Geometry: final body of the model. Coordinates: model frame, mm. A direction names the side the tool comes from. Coordinates: 2 decimals unless noted, no trailing zeros. Write each loop counter-clockwise with the first axis right and the second up, starting at its lowest first coordinate (ties: lowest second). Pieces come first, ordered by that corner, then holes. Notation, with made-up numbers: (-23, 43) -> (-7, 43) arc R32 ccw to (-7, 71) -> close; hole circle Ø1 at (28, 86.5). An arc over 180 degrees is marked (long way). One line per item, written item: value. Start each with the question number.
from build123d import *

# Parameters (mm, degrees)
BOSS_EXTRUDE1_DEPTH = 34.75
SKETCH2_R           = 2
CUT_EXTRUDE1_DEPTH  = 72.445179815
SKETCH3_W           = 30
SKETCH3_H           = 7.896551268
BOSS_EXTRUDE2_DEPTH = 48
SKETCH4_W           = 30
SKETCH4_H           = 6
CUT_EXTRUDE2_DEPTH  = 4
FILLET1_R           = 10
SKETCH5_R           = 9
CUT_EXTRUDE3_DEPTH  = 75.652167363
BOSS_EXTRUDE3_DEPTH = 1
CUT_EXTRUDE4_DEPTH  = 0.5
CUT_EXTRUDE5_START  = -30
CUT_EXTRUDE5_DEPTH  = 30
SKETCH11_W          = 8.25
SKETCH11_H          = 3.125
CUT_EXTRUDE6_DEPTH  = 30


with BuildPart() as part:
    # Sketch1 → Boss-Extrude1 (new body)
    with BuildSketch(Plane(origin=(0, 0, 0), x_dir=(1, 0, 0), z_dir=(0, 1, 0))):
        with BuildLine():
            Line((0, 0), (6.55816832, -13.490382807))
            ThreePointArc((6.55816832, -13.490382807), (30.474828919, -7.985034321), (54.391489518, -13.490382807))
            Line((54.391489518, -13.490382807), (60.949657838, 0))
            ThreePointArc((60.949657838, 0), (30.474828919, 7.014965679), (0, 0))
        make_face()
    extrude(amount=BOSS_EXTRUDE1_DEPTH)

    # Sketch2 → Cut-Extrude1 (cut, through all)
    with BuildSketch(Plane(origin=(0, 34.75, 0), x_dir=(1, 0, 0), z_dir=(0, 1, 0))):
        with Locations(Location((12.974828919, -6.985034321, 0), (0, 0, 270))):
            Circle(SKETCH2_R)
        with Locations(Location((47.974828919, -6.985034321, 0), (0, 0, 90))):
            Circle(SKETCH2_R)
    extrude(amount=-CUT_EXTRUDE1_DEPTH, mode=Mode.SUBTRACT)

    # Sketch3 → Boss-Extrude2 (add)
    with BuildSketch(Plane(origin=(0, 34.75, 0), x_dir=(1, 0, 0), z_dir=(0, 1, 0))):
        with Locations((30.474828919, 8.066690045)):
            Rectangle(SKETCH3_W, SKETCH3_H)
    extrude(amount=-BOSS_EXTRUDE2_DEPTH)

    # Sketch4 → Cut-Extrude2 (cut)
    with BuildSketch(Plane.XY.offset(-4.118414411)):
        with Locations((30.474828919, -3)):
            Rectangle(SKETCH4_W, SKETCH4_H)
    extrude(amount=-CUT_EXTRUDE2_DEPTH, mode=Mode.SUBTRACT)

    # Fillet1
    fillet1_edges = [part.edges().sort_by_distance(p)[0] for p in [
        (15.474828919, -13.25, -8.066690045),
        (45.474828919, -13.25, -8.066690045),
    ]]
    fillet(fillet1_edges, radius=FILLET1_R)

    # Sketch5 → Cut-Extrude3 (cut, through all)
    with BuildSketch(Plane(origin=(0, 0, -12.014965679), x_dir=(-1, 0, 0), z_dir=(0, 0, -1))):
        with Locations((-30.474828919, 19.75)):
            Circle(SKETCH5_R)
    extrude(amount=-CUT_EXTRUDE3_DEPTH, mode=Mode.SUBTRACT)

    # Sketch7 → Boss-Extrude3 (add)
    with BuildSketch(Plane(origin=(0, 0, -12.014965679), x_dir=(-1, 0, 0), z_dir=(0, 0, -1))):
        with BuildLine():
            Line((-21.536068007, 1.453872129), (-26.199769352, 0))
            ThreePointArc((-26.199769352, 0), (-24.751375622, 3.560871216), (-21.536068007, 1.453872129))
        make_face()
        with BuildLine():
            Line((-34.426020337, 3.673663851), (-38.960174422, 5.664158065))
            ThreePointArc((-38.960174422, 5.664158065), (-37.895872331, 1.929105477), (-34.426020337, 3.673663851))
        make_face()
    extrude(amount=BOSS_EXTRUDE3_DEPTH)

    # Sketch8 → Cut-Extrude4 (cut)
    with BuildSketch(Plane(origin=(0, 0, -13.014965679), x_dir=(-1, 0, 0), z_dir=(0, 0, -1))):
        with BuildLine():
            Line((-23.022731531, 0.990416495), (-25.036897729, 0.362516061))
            ThreePointArc((-25.036897729, 0.362516061), (-24.475304572, 2.105499822), (-23.022731531, 0.990416495))
        make_face()
        with BuildLine():
            Line((-35.750767501, 4.255228023), (-37.89390211, 5.196064386))
            ThreePointArc((-37.89390211, 5.196064386), (-37.451768412, 3.29185708), (-35.750767501, 4.255228023))
        make_face()
    extrude(amount=-CUT_EXTRUDE4_DEPTH, mode=Mode.SUBTRACT)

    # Sketch9 → Cut-Extrude5 (cut)
    with BuildSketch(Plane(origin=(0, 34.75, 0), x_dir=(1, 0, 0), z_dir=(0, 1, 0)).offset(CUT_EXTRUDE5_START)):
        with BuildLine():
            Line((30.474828919, 5.014965679), (30.474828919, -7.985034321))
            ThreePointArc((30.474828919, -7.985034321), (37.27763759, -8.409679524), (43.974828919, -9.677022281))
            Line((43.974828919, -9.677022281), (43.974828919, 5.014965679))
            Line((43.974828919, 5.014965679), (30.474828919, 5.014965679))
        make_face()
        with BuildLine():
            ThreePointArc((16.974828919, -9.677022281), (23.672020248, -8.409679524), (30.474828919, -7.985034321))
            Line((30.474828919, -7.985034321), (30.474828919, 5.014965679))
            Line((30.474828919, 5.014965679), (16.974828919, 5.014965679))
            Line((16.974828919, 5.014965679), (16.974828919, -9.677022281))
        make_face()
    extrude(amount=CUT_EXTRUDE5_DEPTH, mode=Mode.SUBTRACT)

    # Sketch11 → Cut-Extrude6 (cut)
    with BuildSketch(Plane(origin=(0, 34.75, 0), x_dir=(1, 0, 0), z_dir=(0, 1, 0))):
        with Locations((12.849828919, -2.547534321)):
            Rectangle(SKETCH11_W, SKETCH11_H)
        with Locations((48.099828919, -2.547534321)):
            Rectangle(SKETCH11_W, SKETCH11_H)
    extrude(amount=-CUT_EXTRUDE6_DEPTH, mode=Mode.SUBTRACT)


solid = part.part
Q1. Cut plane C-C on x = 33. Output: boundary loops of the cut face in (y, z), and give its area (3 significant figures).
Q2. Cut plane B-B on z = 11.25. Output: boundary loops of the cut face in (x, y), and give its area (3 significant figures).
Q3. First-contact query: P1, Ø2.5, axis at x = 48.5, y = 21.5, coming from the -Z side; P2, Ø9, axis at x = 12.5, y = 16.5, coming from the +Z side; P3, Ø10, axis at x = 10, z = -5, coming from the +Y side; P4, Ø15, axis at x = 24, y = 17, coming from the -Z side. Flat tips, straight axial feed; report the tip coordinate or a pass-through.
Q4. Line query: L1, parallel to Z at x = 46.5, y = 14; L2, parallel to X at y = 26, z = 8; L3, parallel to Y at x = 24, z = 6.25. Output: solid intervals per line, ascending. Write a range as from..to.
Q5. Cut plane A-A on y = 25. Output: boundary loops of the cut face in (x, z).
Q6. Cut plane D-D on y = 19.75. Output: boundary loops of the cut face in (x, z), and give its area (3 significant figures).
Q7. Access query for faces 4 (the flat face through (13, 20, 0.985)), 5 (the flat face through (30, 0, 3)), 6 (the flat face through (45.475, 16, -9)), 7 (the flat face through (16.975, 20, -2)). Directions: +Z, -Z, +X, -X, +Y, -Y. A direction counts if a zero-diameter tool reaches every point of the face in a straight line with its end or side. Return the directions, or none.
Q8. Draft query along X for faces 1 (the flat face through (30, -10, -4.118)), 2 (the cylindrical face through (37.952, 1.955, -12.508)), 3 (the flat face through (3.233, 17.132, 6.651)). Return one class per face: pulls with the +X half, pulls with the -X half, needs draft (parallel to the pull), parting line crosses it, or undercut.
Solution:
1. outline: (-13.25, -12.01) -> (11.11, -12.01) -> (11.11, -5.01) -> (4.75, -5.01) -> (4.75, 8.04) -> (0, 8.04) -> (0, -8.12) -> (-6, -8.12) -> (-6, -4.12) -> (-13.25, -4.12) -> close; (28.39, -12.01) -> (34.75, -12.01) -> (34.75, -5.01) -> (28.39, -5.01) -> close
1. area: 265 mm²
2. outline: (5.47, 0) -> (11.86, 0) -> (11.86, 34.75) -> (5.47, 34.75) -> close; (49.09, 0) -> (55.48, 0) -> (55.48, 34.75) -> (49.09, 34.75) -> close
2. area: 444 mm²
3. P1: z = -4.97
3. P2: z = 12.82
3. P3: y = 34.75
3. P4: z = -12.01
4. L1: -5.15..0.99, 4.11..5.63, 8.34..10.38
4. L2: 3.89..11.25, 14.7..16.97, 43.97..46.25, 49.7..57.06
4. L3: 0..4.75
5. outline: (0, 0) arc R69.7 ccw to (15.47, -5.38) -> (15.47, -12.01) -> (23.16, -12.01) -> (23.16, -5.01) -> (16.97, -5.01) -> (16.97, 0.99) -> (8.72, 0.99) -> (8.72, 4.11) -> (16.97, 4.11) -> (16.97, 9.68) arc R54.7 cw to (6.56, 13.49) -> close; (37.78, -12.01) -> (45.47, -12.01) -> (45.47, -5.38) arc R69.7 ccw to (60.95, 0) -> (54.39, 13.49) arc R54.7 cw to (43.97, 9.68) -> (43.97, 4.11) -> (52.22, 4.11) -> (52.22, 0.99) -> (43.97, 0.99) -> (43.97, -5.01) -> (37.78, -5.01) -> close; hole circle Ø4 at (12.97, 6.99); hole circle Ø4 at (47.97, 6.99)
6. outline: (0, 0) arc R69.7 ccw to (15.47, -5.38) -> (15.47, -12.01) -> (21.47, -12.01) -> (21.47, -5.01) -> (16.97, -5.01) -> (16.97, 0.99) -> (8.72, 0.99) -> (8.72, 4.11) -> (16.97, 4.11) -> (16.97, 9.68) arc R54.7 cw to (6.56, 13.49) -> close; (39.47, -12.01) -> (45.47, -12.01) -> (45.47, -5.38) arc R69.7 ccw to (60.95, 0) -> (54.39, 13.49) arc R54.7 cw to (43.97, 9.68) -> (43.97, 4.11) -> (52.22, 4.11) -> (52.22, 0.99) -> (43.97, 0.99) -> (43.97, -5.01) -> (39.47, -5.01) -> close; hole circle Ø4 at (12.97, 6.99); hole circle Ø4 at (47.97, 6.99)
6. area: 442 mm²
7. face 4: +Y
7. face 5: +Z, +X, -X
7. face 6: -Z, +X, +Y, -Y
7. face 7: +Z, +Y
8. face 1: needs draft
8. face 2: undercut
8. face 3: pulls with the -X half
